from build123d import *

# Parameters (mm, degrees)
BOSS_EXTRUDE2_REACH = 139.619
SKETCH6_R           = 4
SKETCH7_R           = 2
CUT_EXTRUDE2_DEPTH  = 5
SKETCH8_R           = 19
CUT_EXTRUDE4_DEPTH  = 83


with BuildPart() as part:
    # Sketch1 → Revolve1 (revolve)
    with BuildSketch(Plane(origin=(0, 0, 0), x_dir=(0, 0, -1), z_dir=(1, 0, 0)), mode=Mode.PRIVATE) as revolve1_sk:
        with BuildLine():
            Line((-22, 130), (-25, 0))
            Line((-25, 0), (-16, 0))
            Line((-16, 0), (-16, 5))
            Line((-16, 5), (-22.884082911, 5))
            Line((-22.884082911, 5), (-20.000532332, 129.953858438))
            Line((-20.000532332, 129.953858438), (-19.998935124, 130.023070781))
            ThreePointArc((-19.998935124, 130.023070781), (-19.698103722, 130.715217023), (-18.99920129, 131))
            Line((-18.99920129, 131), (-16.1975525, 131))
            Line((-16.1975525, 131), (0, 131))
            Line((0, 131), (0, 133))
            Line((0, 133), (-16.1975525, 133))
            Line((-16.1975525, 133), (-18.99920129, 133))
            ThreePointArc((-18.99920129, 133), (-21.095908586, 132.14565107), (-21.998402792, 130.069212342))
            Line((-21.998402792, 130.069212342), (-22, 130))
        make_face()
    revolve(revolve1_sk.sketch.rotate(Axis((0, 0, 0), (0, 1, 0)), 180), axis=Axis((0, 0, 0), (0, 1, 0)))

    # Sketch6 → Boss-Extrude2 (add, up to next)
    with BuildSketch(Plane.XZ, mode=Mode.PRIVATE) as boss_extrude2_sk1:
        with Locations((0, 20.5)):
            Circle(SKETCH6_R)
    boss_extrude2_tool1 = extrude(boss_extrude2_sk1.sketch, amount=-BOSS_EXTRUDE2_REACH, mode=Mode.PRIVATE) - part.part
    # Sketch6 → Boss-Extrude2 (add, up to next)
    with BuildSketch(Plane.XZ, mode=Mode.PRIVATE) as boss_extrude2_sk2:
        with Locations((17.753520778, -10.25)):
            Circle(SKETCH6_R)
    boss_extrude2_tool2 = extrude(boss_extrude2_sk2.sketch, amount=-BOSS_EXTRUDE2_REACH, mode=Mode.PRIVATE) - part.part
    # Sketch6 → Boss-Extrude2 (add, up to next)
    with BuildSketch(Plane.XZ, mode=Mode.PRIVATE) as boss_extrude2_sk3:
        with Locations((-17.753520778, -10.25)):
            Circle(SKETCH6_R)
    boss_extrude2_tool3 = extrude(boss_extrude2_sk3.sketch, amount=-BOSS_EXTRUDE2_REACH, mode=Mode.PRIVATE) - part.part
    add(boss_extrude2_tool1.solids().sort_by_distance((0, 0, 20.5))[0])
    add(boss_extrude2_tool2.solids().sort_by_distance((17.753521, 0, -10.25))[0])
    add(boss_extrude2_tool3.solids().sort_by_distance((-17.753521, 0, -10.25))[0])

    # Sketch7 → Cut-Extrude2 (cut)
    with BuildSketch(Plane.XZ):
        with Locations(Location((0, 20.5, 0), (0, 0, 270))):
            Circle(SKETCH7_R)
        with Locations(Location((17.753520778, -10.25, 0), (0, 0, 270))):
            Circle(SKETCH7_R)
        with Locations(Location((-17.753520778, -10.25, 0), (0, 0, 270))):
            Circle(SKETCH7_R)
    extrude(amount=-CUT_EXTRUDE2_DEPTH, mode=Mode.SUBTRACT)

    # Sketch8 → Cut-Extrude4 (cut)
    with BuildSketch(Plane(origin=(0, 48, 0), x_dir=(-1, 0, 0), z_dir=(0, -1, 0))):
        Circle(SKETCH8_R)
    extrude(amount=-CUT_EXTRUDE4_DEPTH, mode=Mode.SUBTRACT)


solid = part.part
Work out the finished part from the listing and answer in its coordinate system (mm). A direction names the side the tool comes from. Round coordinates to 2 decimals unless told otherwise and drop trailing zeros. Loops run counter-clockwise (first coordinate to the right, second up) from the corner with the lowest first, then second, coordinate; pieces in that order, holes last. Notation, with made-up numbers: (1.25, 10.25) -> (54.25, 10.25) arc R25 cw to (54.25, 24.25) -> close; hole circle Ø4 at (64.5, 64). An arc over 180 degrees is marked (long way). Use one line per item in the form item = value.
(1) A tool of negligible diameter and unlimited length cuts with its end or side. For faces 4 (the cylindrical face through (-15.77, 2.46, -9.99)), 5 (the flat face through (-13.7, 5, -8.7)), 6 (the flat face through (16.3, 0, 0.3)), from which of +Z, -Z, +X, -X, +Y, -Y can it reach the whole face along a straight path? Write none if from no direction.
Answer list:
face_4 = -Y
face_5 = none
face_6 = +Z, -Z, +X, -X, -Y
(2) Find section A-A on y = 53. Give the vertices of the cut face in (x, z).
Answer list:
outline = circle Ø47.55 at (0, 0); hole (-20.5, -7.34) arc R4 cw to (-17.94, -6.25) arc R19 ccw to (-14.39, -12.41) arc R4 cw to (-16.61, -14.08) arc R21.78 ccw to (16.61, -14.08) arc R4 cw to (14.39, -12.41) arc R19 ccw to (17.94, -6.25) arc R4 cw to (20.5, -7.34) arc R21.78 ccw to (3.89, 21.43) arc R4 cw to (3.55, 18.66) arc R19 ccw to (-3.55, 18.66) arc R4 cw to (-3.89, 21.43) arc R21.78 ccw to start
(3) Flat-ended cylindrical pins translate along their axes: P1, Ø4, axis at x = -17, y = 48, coming from the +Z side; P2, Ø19, axis at x = -2, z = 6, coming from the -Y side; P3, Ø3, axis at x = 0, z = 20.5, coming from the -Y side; P4, Ø5, axis at x = -17.75, z = -10.25, coming from the +Y side. Find the tip coordinate at first contact, or state that the pin passes through.
Answer list:
P1 = 18.6
P2 = 131
P3 = 5
P4 = 133
(4) For a pull along Y with two mould halves and no side action, classify faces 1 (the cylindrical face through (-14.231, 39.118, -8.354)), 2 (the flat face through (0, 133, 0)), 3 (the flat face through (18, 5, -10)) as released by +Y, released by -Y, zero draft, split by the parting line, or undercut.
Answer list:
face_1 = undercut
face_2 = released by +Y
face_3 = released by -Y
(5) Straight lines are drawn through the part: line 1 (X direction, y = 1, z = 0); line 2 (X direction, y = 8, z = -8); line 3 (Y direction, x = 12, z = -11.5). For each, find the intervals that lie inside material, in ascending order.
Answer list:
line_1 = -24.98 to -16, 16 to 24.98
line_2 = -23.49 to -21.37, -21.06 to -14.45, 14.45 to 21.06, 21.37 to 23.49
line_3 = 0 to 5, 131 to 133
(6) Find section B-B on y = 15.5. Give the vertices of the cut face in (x, z).
Answer list:
outline = circle Ø49.28 at (0, 0); hole (-21.14, -8.12) arc R4 cw (long way) to (-17.6, -14.25) arc R22.64 ccw to (17.6, -14.25) arc R4 cw (long way) to (21.14, -8.12) arc R22.64 ccw to (3.54, 22.36) arc R4 cw (long way) to (-3.54, 22.36) arc R22.64 ccw to start
